Read the model definition and answer for the solid it produces. Units are mm, in the model's axes. A direction names the side the tool comes from. Coordinates: 2 decimals unless noted, no trailing zeros. Order: outer loops, then holes, each group sorted by start corner. A loop starts at its lowest first (then second) coordinate and runs counter-clockwise, first axis right, second up. Notation, with made-up numbers: M 30.5,34 L 36.5,34 A21 ccw 36.5,51 Z; hole C 33,34.5 d10. An arc over 180 degrees is marked long. Use a Markdown table: item, result. Add a question column.
1) Find the intervals of material crossed by probe 1 along X at (y, z) = (18.5, 17.5); probe 2 along X at (y, z) = (23, 29), in increasing order. Write a range as [from, to].
2) The mould has two halves that part along X. Classify faces 1 (the face through (27.85, -27.89, 14.45)), 2 (the face through (-28.75, 0, 14)), 3 (the face through (-25.75, 0, 16)): released by +X, released by -X, zero draft, split by the parting line, or undercut.
3) Each of these flat-tipped pins is pushed along its axis until it touches: pin 1 Ø1.6 at (x, z) = (-26.5, 30.5) entering from +Y; pin 2 Ø5 at (x, y) = (22, -13) entering from +Z; pin 3 Ø1.6 at (x, z) = (-26.5, 30.5) entering from -Y. Where does it stop, or does it pass through?
4) Find section D-D on y = 4. Write down the section's boundary in (x, z).
5) Find section B-B on z = 11. Write down the section's boundary in (x, y).
6) For faces 4 (the face through (0, -27.2, 30)), 5 (the face through (25.75, 0, 16)), 6 (the face through (27.2, 0, 30)), determine the directions among +Z, -Z, +X, -X, +Y, -Y from which every point of the face is accessible in a straight line to the end or side of a thin tool.
7) Find section A-A on x = 13.5. Write down the section's boundary in (y, z), plus the area to 3 significant figures.
from build123d import *

# Parameters (mm, degrees)
SKETCH_W        = 57.5
SKETCH_H        = 57.5
PAD_DEPTH       = 1.5
SKETCH001_W     = 57.5
SKETCH001_H     = 57.5
SKETCH001_W_2   = 51.5
SKETCH001_H_2   = 51.5
PAD001_DEPTH    = 30
SKETCH002_W     = 57.5
SKETCH002_H     = 57.5
SKETCH002_W_2   = 54.4
SKETCH002_H_2   = 54.4
POCKET_DEPTH    = 3
FILLET_R        = 3
SKETCH003_W     = 10
SKETCH003_H     = 3
POCKET001_DEPTH = 5


with BuildPart() as part:
    # Sketch → Pad (new body)
    with BuildSketch(Plane.XY):
        Rectangle(SKETCH_W, SKETCH_H)
    extrude(amount=PAD_DEPTH)

    # Sketch001 (on Face6 of Pad) → Pad001 (join)
    with BuildSketch(Plane.XY.offset(1.5)):
        Rectangle(SKETCH001_W, SKETCH001_H)
        Rectangle(SKETCH001_W_2, SKETCH001_H_2, mode=Mode.SUBTRACT)
    extrude(amount=PAD001_DEPTH)

    # Sketch002 (on Face9 of Pad001) → Pocket (cut)
    with BuildSketch(Plane.XY.offset(31.5)):
        Rectangle(SKETCH002_W, SKETCH002_H)
        Rectangle(SKETCH002_W_2, SKETCH002_H_2, mode=Mode.SUBTRACT)
    extrude(amount=-POCKET_DEPTH, mode=Mode.SUBTRACT)

    # Fillet
    fillet_edges = [part.edges().sort_by_distance(p)[0] for p in [
        (-28.75, 28.75, 15),
        (-28.75, 28.75, 0.75),
        (-28.75, -28.75, 0.75),
        (-28.75, -28.75, 15),
        (28.75, -28.75, 0.75),
        (28.75, -28.75, 15),
        (28.75, 28.75, 15),
        (28.75, 28.75, 0.75),
    ]]
    fillet(fillet_edges, radius=FILLET_R)

    # Sketch003 (on Face22 of Fillet) → Pocket001 (cut)
    with BuildSketch(Plane(origin=(-27.2, 0, 0), x_dir=(0, -1, 0), z_dir=(-1, 0, 0))):
        with Locations((0, 30)):
            Rectangle(SKETCH003_W, SKETCH003_H)
    extrude(amount=-POCKET001_DEPTH, mode=Mode.SUBTRACT)


solid = part.part
Check result:
| question | item | result |
|---|---|---|
| 1 | probe 1 | x = [-28.75, -25.75], [25.75, 28.75] |
| 1 | probe 2 | x = [-27.2, -25.75], [25.75, 27.2] |
| 2 | face 1 | released by +X |
| 2 | face 2 | released by -X |
| 2 | face 3 | undercut |
| 3 | pin 1 | stops at y = 27.2 |
| 3 | pin 2 | stops at z = 1.5 |
| 3 | pin 3 | stops at y = -27.2 |
| 4 | outline | M -28.75,0 L 28.75,0 L 28.75,28.5 L 27.2,28.5 L 27.2,31.5 L 25.75,31.5 L 25.75,1.5 L -25.75,1.5 L -25.75,28.5 L -28.75,28.5 Z |
| 5 | outline | M -28.75,-25.75 A3 ccw -25.75,-28.75 L 25.75,-28.75 A3 ccw 28.75,-25.75 L 28.75,25.75 A3 ccw 25.75,28.75 L -25.75,28.75 A3 ccw -28.75,25.75 Z; hole M -25.75,-25.75 L 25.75,-25.75 L 25.75,25.75 L -25.75,25.75 Z |
| 6 | face 4 | +Z, +X, -X, -Y |
| 6 | face 5 | +Z |
| 6 | face 6 | +Z, +X, +Y, -Y |
| 7 | outline | M -28.75,0 L 28.75,0 L 28.75,28.5 L 27.2,28.5 L 27.2,31.5 L 25.75,31.5 L 25.75,1.5 L -25.75,1.5 L -25.75,31.5 L -27.2,31.5 L -27.2,28.5 L -28.75,28.5 Z |
| 7 | area | 257 mm2 |
